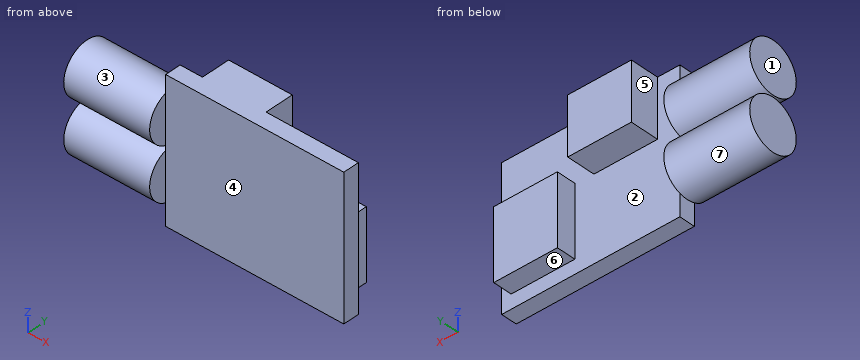
from build123d import *

# Parameters (mm, degrees)
SKETCH1_W           = 28
SKETCH1_H           = 22
BOSS_EXTRUDE1_DEPTH = 2.5
SKETCH2_W           = 10
SKETCH2_H           = 9
BOSS_EXTRUDE2_DEPTH = 4.5
SKETCH3_W           = 10
SKETCH3_H           = 11
BOSS_EXTRUDE3_DEPTH = 3
SKETCH4_R           = 4
BOSS_EXTRUDE4_DEPTH = 13.5


with BuildPart() as part:
    # Sketch1 → Boss-Extrude1 (new body)
    with BuildSketch(Plane(origin=(0, 0, 0), x_dir=(1, 0, 0), z_dir=(0, 1, 0))):
        Rectangle(SKETCH1_W, SKETCH1_H)
    extrude(amount=BOSS_EXTRUDE1_DEPTH)

    # Sketch2 → Boss-Extrude2 (add)
    with BuildSketch(Plane(origin=(0, 2.5, 0), x_dir=(1, 0, 0), z_dir=(0, 1, 0))):
        with Locations((-5.5, -6.5)):
            Rectangle(SKETCH2_W, SKETCH2_H)
    extrude(amount=BOSS_EXTRUDE2_DEPTH)

    # Sketch3 → Boss-Extrude3 (add)
    with BuildSketch(Plane(origin=(0, 2.5, 0), x_dir=(1, 0, 0), z_dir=(0, 1, 0))):
        with Locations((7.5, 3.3)):
            Rectangle(SKETCH3_W, SKETCH3_H)
    extrude(amount=BOSS_EXTRUDE3_DEPTH)

    # Sketch4 → Boss-Extrude4 (add)
    with BuildSketch(Plane.ZY.offset(14)):
        with Locations((-3.8, 1.25)):
            Circle(SKETCH4_R)
        with Locations((4.5, 1.25)):
            Circle(SKETCH4_R)
    extrude(amount=BOSS_EXTRUDE4_DEPTH)


solid = part.part
Work out the finished part from the listing and answer in its coordinate system (mm). Face numbers are marked on the shaded views. A direction names the side the tool comes from. Round coordinates to 2 decimals unless told otherwise and drop trailing zeros. Write each loop counter-clockwise with the first axis right and the second up, starting at its lowest first coordinate (ties: lowest second). Pieces come first, ordered by that corner, then holes.
1) Given pin 1 Ø2 at (y, z) = (-1.5, -3) entering from +X; pin 2 Ø2.5 at (x, y) = (6.5, 4.5) entering from -Z; pin 3 Ø11 at (x, z) = (-6.5, -2.5) entering from -Y, each flat-ended and moving along its own axis, determine where each tip first touches the part or whether it passes through.
2) A cutting plane is placed at D-D (y = 1.25). Give the vertices of the cut face in (x, z).
3) A tool of negligible diameter and unlimited length cuts with its end or side. For the marked faces 4, 5, 6 and 7, from which of +Z, -Z, +X, -X, +Y, -Y can it reach the whole face along a straight path? Write none if from no direction.
4) A cutting plane is placed at A-A (z = -3.8). Give the vertices of the cut face in (x, y).
5) A cutting plane is placed at C-C (x = -23). Give the vertices of the cut face in (y, z).
6) The mould has two halves that part along X. Classify the marked faces 1, 2 and 3: pulls with the +X half, pulls with the -X half, needs draft (parallel to the pull), parting line crosses it, or undercut.
7) A cutting plane is placed at B-B (x = 4). Give the vertices of the cut face in (y, z).
8) Straight lines are drawn through the part: line 1 (X direction, y = 2.75, z = -2); line 2 (X direction, y = 3, z = 5.5); line 3 (Y direction, x = 1, z = 9.5). For each, find the intervals that lie inside material, in ascending order.
Completed:
1. pin 1: stops at x = -14
1. pin 2: stops at z = -8.8
1. pin 3: stops at y = 0
2. outline: (-27.5, -7.8) - (-14, -7.8) - (-14, -11) - (14, -11) - (14, 11) - (-14, 11) - (-14, 8.5) - (-27.5, 8.5) - (-27.5, 0.5) - (-14, 0.5) - (-14, 0.2) - (-27.5, 0.2) - close
3. face 4: +Z, -Z, +X, -Y
3. face 5: +Z, -Z, +Y
3. face 6: -Z, +X, -X, +Y
3. face 7: -X
4. outline: (-27.5, -2.75) - (-14, -2.75) - (-14, 0) - (14, 0) - (14, 2.5) - (12.5, 2.5) - (12.5, 5.5) - (2.5, 5.5) - (2.5, 2.5) - (-14, 2.5) - (-14, 5.25) - (-27.5, 5.25) - close
5. outline: circle Ø8 at (1.25, -3.8); circle Ø8 at (1.25, 4.5)
6. face 1: pulls with the -X half
6. face 2: undercut
6. face 3: needs draft
7. outline: (0, -11) - (2.5, -11) - (2.5, -8.8) - (5.5, -8.8) - (5.5, 2.2) - (2.5, 2.2) - (2.5, 11) - (0, 11) - close
8. line 1: x = -27.5 to -14, 2.5 to 12.5
8. line 2: x = -27.5 to -14, -10.5 to -0.5
8. line 3: y = 0 to 2.5
